Build history of the part. All positions in model axes, mm. A direction names the side the tool comes from. Give positions to 0.01 mm unless a question says otherwise; leave off trailing zeros. Write each loop counter-clockwise with the first axis right and the second up, starting at its lowest first coordinate (ties: lowest second). Pieces come first, ordered by that corner, then holes.
from build123d import *

# Parameters (mm, degrees)
F0_W     = 233
F0_H     = 81
F0_W_2   = 227.4
F0_H_2   = 75.4
F1_DEPTH = 8.8
F2_W     = 10
F2_H     = 4.4
F3_DEPTH = 25
F4_W     = 10
F4_H     = 1.2
F5_DEPTH = 2.4


with BuildPart() as f1:
    # F0 (on Top) → F1 (new body)
    with BuildSketch(Plane.XY):
        Rectangle(F0_W, F0_H)
        Rectangle(F0_W_2, F0_H_2, mode=Mode.SUBTRACT)
    extrude(amount=F1_DEPTH)

    # F2 (on face) → F3 (cut)
    with BuildSketch(Plane(origin=(0, 40.5, 0), x_dir=(-1, 0, 0), z_dir=(0, 1, 0))):
        with Locations((76.5, 2.2)):
            Rectangle(F2_W, F2_H)
    extrude(amount=-F3_DEPTH, mode=Mode.SUBTRACT)

    # F4 (on face) → F5 (cut)
    with BuildSketch(Plane(origin=(0, 0, 4.4), x_dir=(1, 0, 0), z_dir=(0, 0, -1))):
        with Locations((-76.5, -38.3)):
            Rectangle(F4_W, F4_H)
    extrude(amount=-F5_DEPTH, mode=Mode.SUBTRACT)


solid = f1.part
1. Drop flat-ended pins along their axis: pin 1 (0.8 mm diameter, centred on x = -76, y = 40, fed in from -Z); pin 2 (0.6 mm diameter, centred on x = -77, y = 38, fed in from -Z). Give the stop position or say it passes through.
2. 3-axis set-ups, long thin cutter, end or side, ignore diameter. For faces 5 (the face through (-2, 40.5, 4)), 6 (the face through (-2, 37.7, 4)): which of +Z, -Z, +X, -X, +Y, -Y reach the whole face in a straight line?
3. Drill centre lines: line 1 along Y through (x, z) = (5, 2.5); line 2 along X through (y, z) = (25, 5.75); line 3 along Y through (x, z) = (-81, 2.25). Where is each one in solid material? Low to high.
4. Saw through at C-C on z = 1.5. Give the cut face in (x, y).
5. Mould opens along X. For faces 1 (the face through (116.5, -1, 4)), 2 (the face through (-1, -39, 0)), 3 (the face through (-113.7, -1, 4)), 4 (the face through (113.7, -1, 4)) say: pulls with the +X half, pulls with the -X half, needs draft (parallel to the pull), parting line crosses it, or undercut.
6. Saw through at B-B on x = -44. Give the cut face in (y, z).
7. Saw through at A-A on y = 2. Give the cut face in (x, z), plus the area to 3 significant figures.
Outcome:
1. pin 1: stops at z = 4.4
1. pin 2: stops at z = 6.8
2. face 5: +Z, -Z, +X, -X, +Y
2. face 6: +Z, -Z
3. line 1: y = -40.5 to -37.7, 37.7 to 40.5
3. line 2: x = -116.5 to -113.7, 113.7 to 116.5
3. line 3: y = -40.5 to -37.7
4. outline: (-116.5, -40.5) - (116.5, -40.5) - (116.5, 40.5) - (-71.5, 40.5) - (-71.5, 37.7) - (113.7, 37.7) - (113.7, -37.7) - (-113.7, -37.7) - (-113.7, 37.7) - (-81.5, 37.7) - (-81.5, 40.5) - (-116.5, 40.5) - close
5. face 1: pulls with the +X half
5. face 2: needs draft
5. face 3: undercut
5. face 4: undercut
6. outline: (-40.5, 0) - (-37.7, 0) - (-37.7, 8.8) - (-40.5, 8.8) - close; (37.7, 0) - (40.5, 0) - (40.5, 8.8) - (37.7, 8.8) - close
7. outline: (-116.5, 0) - (-113.7, 0) - (-113.7, 8.8) - (-116.5, 8.8) - close; (113.7, 0) - (116.5, 0) - (116.5, 8.8) - (113.7, 8.8) - close
7. area: 49.3 mm2
